Work out the finished part from the listing and answer in its coordinate system (mm). A direction names the side the tool comes from. Round coordinates to 2 decimals unless told otherwise and drop trailing zeros. Write each loop counter-clockwise with the first axis right and the second up, starting at its lowest first coordinate (ties: lowest second). Pieces come first, ordered by that corner, then holes.
1. Find section D-D (y = -35.5). Write down the section's boundary in (x, z), and give its area (3 significant figures).
2. Determine the mould class of faces 1 (the face through (4, -10, -2)), 2 (the face through (2, -25, 14)), 3 (the face through (1, -37, 7)) for opening direction Z: pulls with the +Z half, pulls with the -Z half, needs draft (parallel to the pull), parting line crosses it, or undercut.
3. Straight lines are drawn through the part: probe 1 along Y at (x, z) = (0.4, 7); probe 2 along Z at (x, y) = (2, -39); probe 3 along X at (y, z) = (-38, 2). For each, find the intervals that lie inside material, in ascending order.
4. Find section A-A (y = -43). Write down the section's boundary in (x, z).
5. A tool of negligible diameter and unlimited length cuts with its end or side. For faces 4 (the face through (8, -20, 4)), 5 (the face through (2, -25, 0)), 6 (the face through (2, -37, 0.65)), 7 (the face through (8, -10, 7)), from which of +Z, -Z, +X, -X, +Y, -Y can it reach the whole face along a straight path? Write none if from no direction.
6. Flat-ended cylindrical pins translate along their axes: pin 1 Ø2 at (y, z) = (-20, -1.5) entering from -X; pin 2 Ø1.5 at (x, z) = (2, 7) entering from -Y; pin 3 Ø1.5 at (x, y) = (3, -23.5) entering from -Z; pin 4 Ø8 at (y, z) = (-31, 7) entering from +X. Find the tip coordinate at first contact, or state that the pin passes through.
7. Find section C-C (z = 1.25). Write down the section's boundary in (x, y), and give its area (4 significant figures).
8. Find section B-B (z = 6.5). Write down the section's boundary in (x, y), and give its area (3 significant figures).
```python
from build123d import *

# Parameters (mm, degrees)
CROQUIS1_W              = 14
CROQUIS1_H              = 50
SALIENTE_EXTRUIR1_DEPTH = 4
CROQUIS2_W              = 3
CROQUIS2_H              = 12.7
CORTAR_EXTRUIR1_DEPTH   = 26.5
SALIENTE_EXTRUIR2_DEPTH = 7.1
CORTAR_EXTRUIR2_REACH   = 54.896
CROQUIS4_R              = 3


with BuildPart() as part:
    # Croquis1 → Saliente-Extruir1 (new body)
    with BuildSketch(Plane(origin=(0, 0, 0), x_dir=(0, 0, -1), z_dir=(1, 0, 0))):
        with Locations((-7, -25)):
            Rectangle(CROQUIS1_W, CROQUIS1_H)
    extrude(amount=SALIENTE_EXTRUIR1_DEPTH)

    # Croquis2 → Cortar-Extruir1 (cut)
    with BuildSketch(Plane.XZ.offset(50)):
        with Locations((2.5, 7)):
            Rectangle(CROQUIS2_W, CROQUIS2_H)
    extrude(amount=-CORTAR_EXTRUIR1_DEPTH, mode=Mode.SUBTRACT)

    # Croquis3 → Saliente-Extruir2 (add)
    with BuildSketch(Plane(origin=(4, 0, 0), x_dir=(0, 0, -1), z_dir=(1, 0, 0))):
        with BuildLine():
            ThreePointArc((0, -20), (4, -10), (0, 0))
            Line((0, 0), (0, -10))
            Line((0, -10), (0, -20))
        make_face()
        Polygon((0, 0), (-7, 0), (-7, -20), (0, -20), (0, -10), align=None)
    extrude(amount=SALIENTE_EXTRUIR2_DEPTH)

    # Croquis4 → Cortar-Extruir2 (cut, up to next)
    with BuildSketch(Plane(origin=(1, 0, 0), x_dir=(0, 0, -1), z_dir=(1, 0, 0)), mode=Mode.PRIVATE) as cortar_extruir2_sk1:
        with Locations((-7, -31)):
            Circle(CROQUIS4_R)
    cortar_extruir2_tool1 = extrude(cortar_extruir2_sk1.sketch, amount=-CORTAR_EXTRUIR2_REACH, mode=Mode.PRIVATE) & part.part
    # Croquis4 → Cortar-Extruir2 (cut, up to next)
    with BuildSketch(Plane(origin=(1, 0, 0), x_dir=(0, 0, -1), z_dir=(1, 0, 0)), mode=Mode.PRIVATE) as cortar_extruir2_sk2:
        with Locations((-7, -43)):
            Circle(CROQUIS4_R)
    cortar_extruir2_tool2 = extrude(cortar_extruir2_sk2.sketch, amount=-CORTAR_EXTRUIR2_REACH, mode=Mode.PRIVATE) & part.part
    add(cortar_extruir2_tool1.solids().sort_by_distance((1, -31, 7))[0], mode=Mode.SUBTRACT)
    add(cortar_extruir2_tool2.solids().sort_by_distance((1, -43, 7))[0], mode=Mode.SUBTRACT)


solid = part.part
```
Worked answers:
1. outline: (0, 0) - (4, 0) - (4, 0.65) - (1, 0.65) - (1, 13.35) - (4, 13.35) - (4, 14) - (0, 14) - close
1. area: 17.9 mm2
2. face 1: needs draft
2. face 2: pulls with the +Z half
2. face 3: undercut
3. probe 1: y = -50 to -46, -40 to -34, -28 to 0
3. probe 2: z = 0 to 0.65, 13.35 to 14
3. probe 3: x = 0 to 1
4. outline: (0, 0) - (4, 0) - (4, 0.65) - (1, 0.65) - (1, 4) - (0, 4) - close; (0, 10) - (1, 10) - (1, 13.35) - (4, 13.35) - (4, 14) - (0, 14) - close
5. face 4: +Z, -Z, +X, -Y
5. face 5: -Z, -X, +Y, -Y
5. face 6: +X, -Y
5. face 7: +Z, +X, +Y, -Y
6. pin 1: passes through
6. pin 2: stops at y = -23.5
6. pin 3: stops at z = 0
6. pin 4: stops at x = 1
7. outline: (0, -50) - (1, -50) - (1, -23.5) - (4, -23.5) - (4, -20) - (11.1, -20) - (11.1, 0) - (0, 0) - close
7. area: 262.5 mm2
8. outline: (0, -50) - (1, -50) - (1, -45.96) - (0, -45.96) - close; (0, -40.04) - (1, -40.04) - (1, -33.96) - (0, -33.96) - close; (0, -28.04) - (1, -28.04) - (1, -23.5) - (4, -23.5) - (4, -20) - (11.1, -20) - (11.1, 0) - (0, 0) - close
8. area: 251 mm2
